CAD build for the part. Positions are in the model's coordinates, mm. Face numbers are marked on the shaded views. Give positions to 0.01 mm unless a question says otherwise; leave off trailing zeros. Write each loop counter-clockwise with the first axis right and the second up, starting at its lowest first coordinate (ties: lowest second). Pieces come first, ordered by that corner, then holes. Notation, with made-up numbers: (-19.75, 19) - (-15.75, 19) arc R33 ccw to (-15.75, 53) - close; hole circle Ø5 at (76, -8). An arc over 180 degrees is marked (long way). Answer as a JSON object with one key per item and string values.
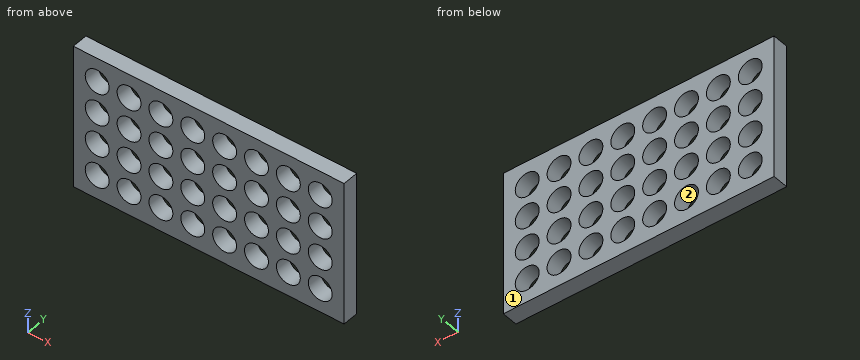
from build123d import *

# Parameters (mm, degrees)
SKETCH1_W           = 68
SKETCH1_H           = 36
SKETCH1_R           = 3
BOSS_EXTRUDE1_DEPTH = 4


with BuildPart() as part:
    # Sketch1 → Boss-Extrude1 (new body)
    with BuildSketch(Plane(origin=(0, 0, 0), x_dir=(1, 0, 0), z_dir=(0, 1, 0))):
        with Locations((34, 18)):
            Rectangle(SKETCH1_W, SKETCH1_H)
        with Locations(Location((6, 6, 0), (0, 0, 270))):
            Circle(SKETCH1_R, mode=Mode.SUBTRACT)
        with Locations(Location((14, 6, 0), (0, 0, 270))):
            Circle(SKETCH1_R, mode=Mode.SUBTRACT)
        with Locations(Location((22, 6, 0), (0, 0, 270))):
            Circle(SKETCH1_R, mode=Mode.SUBTRACT)
        with Locations(Location((30, 6, 0), (0, 0, 270))):
            Circle(SKETCH1_R, mode=Mode.SUBTRACT)
        with Locations(Location((38, 6, 0), (0, 0, 270))):
            Circle(SKETCH1_R, mode=Mode.SUBTRACT)
        with Locations(Location((46, 6, 0), (0, 0, 270))):
            Circle(SKETCH1_R, mode=Mode.SUBTRACT)
        with Locations(Location((54, 6, 0), (0, 0, 270))):
            Circle(SKETCH1_R, mode=Mode.SUBTRACT)
        with Locations(Location((62, 6, 0), (0, 0, 270))):
            Circle(SKETCH1_R, mode=Mode.SUBTRACT)
        with Locations(Location((14, 14, 0), (0, 0, 270))):
            Circle(SKETCH1_R, mode=Mode.SUBTRACT)
        with Locations(Location((22, 14, 0), (0, 0, 270))):
            Circle(SKETCH1_R, mode=Mode.SUBTRACT)
        with Locations(Location((30, 14, 0), (0, 0, 270))):
            Circle(SKETCH1_R, mode=Mode.SUBTRACT)
        with Locations(Location((38, 14, 0), (0, 0, 270))):
            Circle(SKETCH1_R, mode=Mode.SUBTRACT)
        with Locations(Location((46, 14, 0), (0, 0, 270))):
            Circle(SKETCH1_R, mode=Mode.SUBTRACT)
        with Locations(Location((54, 14, 0), (0, 0, 270))):
            Circle(SKETCH1_R, mode=Mode.SUBTRACT)
        with Locations(Location((62, 14, 0), (0, 0, 270))):
            Circle(SKETCH1_R, mode=Mode.SUBTRACT)
        with Locations(Location((14, 22, 0), (0, 0, 270))):
            Circle(SKETCH1_R, mode=Mode.SUBTRACT)
        with Locations(Location((22, 22, 0), (0, 0, 270))):
            Circle(SKETCH1_R, mode=Mode.SUBTRACT)
        with Locations(Location((30, 22, 0), (0, 0, 270))):
            Circle(SKETCH1_R, mode=Mode.SUBTRACT)
        with Locations(Location((38, 22, 0), (0, 0, 270))):
            Circle(SKETCH1_R, mode=Mode.SUBTRACT)
        with Locations(Location((46, 22, 0), (0, 0, 270))):
            Circle(SKETCH1_R, mode=Mode.SUBTRACT)
        with Locations(Location((54, 22, 0), (0, 0, 270))):
            Circle(SKETCH1_R, mode=Mode.SUBTRACT)
        with Locations(Location((62, 22, 0), (0, 0, 270))):
            Circle(SKETCH1_R, mode=Mode.SUBTRACT)
        with Locations(Location((14, 30, 0), (0, 0, 270))):
            Circle(SKETCH1_R, mode=Mode.SUBTRACT)
        with Locations(Location((22, 30, 0), (0, 0, 270))):
            Circle(SKETCH1_R, mode=Mode.SUBTRACT)
        with Locations(Location((30, 30, 0), (0, 0, 270))):
            Circle(SKETCH1_R, mode=Mode.SUBTRACT)
        with Locations(Location((38, 30, 0), (0, 0, 270))):
            Circle(SKETCH1_R, mode=Mode.SUBTRACT)
        with Locations(Location((46, 30, 0), (0, 0, 270))):
            Circle(SKETCH1_R, mode=Mode.SUBTRACT)
        with Locations(Location((54, 30, 0), (0, 0, 270))):
            Circle(SKETCH1_R, mode=Mode.SUBTRACT)
        with Locations(Location((62, 30, 0), (0, 0, 270))):
            Circle(SKETCH1_R, mode=Mode.SUBTRACT)
        with Locations(Location((6, 14, 0), (0, 0, 270))):
            Circle(SKETCH1_R, mode=Mode.SUBTRACT)
        with Locations(Location((6, 22, 0), (0, 0, 270))):
            Circle(SKETCH1_R, mode=Mode.SUBTRACT)
        with Locations(Location((6, 30, 0), (0, 0, 270))):
            Circle(SKETCH1_R, mode=Mode.SUBTRACT)
    extrude(amount=BOSS_EXTRUDE1_DEPTH)


solid = part.part
Item 1: Cut at A-A (x = 6). Give the cut face in (y, z), and give its area (3 significant figures).
Entries:
{"outline": "(0, -36) - (4, -36) - (4, -33) - (0, -33) - close; (0, -27) - (4, -27) - (4, -25) - (0, -25) - close; (0, -19) - (4, -19) - (4, -17) - (0, -17) - close; (0, -11) - (4, -11) - (4, -9) - (0, -9) - close; (0, -3) - (4, -3) - (4, 0) - (0, 0) - close", "area": "48.0 mm2"}
Item 2: Probe line 1 (Z direction, x = 13, y = 2.9); line 2 (Z direction, x = 12, y = 1.8). List the from-to ranges inside material, lowest first. Write a range as from..to.
Entries:
{"line 1": "-36..-32.83, -27.17..-24.83, -19.17..-16.83, -11.17..-8.83, -3.17..0", "line 2": "-36..-32.24, -27.76..-24.24, -19.76..-16.24, -11.76..-8.24, -3.76..0"}
Item 3: Mould opens along X. For the marked faces 1 and 2 say: +X half, -X half, draft (parallel to the pull), parting line (faces both ways), or undercut.
Entries:
{"face 1": "draft", "face 2": "undercut"}
Item 4: Cut at B-B (z = -6). State how many separate pieces and enclosed holes the cut face has, and give its area (3 significant figures).
Entries:
{"separate pieces": "9", "enclosed holes": "0", "area": "80.0 mm2"}
